```python
from build123d import *

# Parameters (mm, degrees)
SKETCH1_W           = 56
SKETCH1_H           = 100
BOSS_EXTRUDE1_DEPTH = 1.5
SKETCH2_W           = 20
SKETCH2_H           = 5.05
BOSS_EXTRUDE2_DEPTH = 10
SKETCH3_W           = 13.1
SKETCH3_H           = 13.1
CUT_EXTRUDE1_DEPTH  = 112.005866962
BOSS_EXTRUDE3_DEPTH = 5
BOSS_EXTRUDE4_DEPTH = 5
SKETCH6_W           = 7
SKETCH6_H           = 1.5
SKETCH6_W_2         = 1.5
SKETCH6_H_2         = 7
BOSS_EXTRUDE5_DEPTH = 4
SKETCH7_W           = 15
SKETCH7_H           = 1.3
CUT_EXTRUDE2_DEPTH  = 112.005866962
SKETCH8_W           = 13.4
SKETCH8_H           = 8.5
SKETCH8_W_2         = 10
SKETCH8_H_2         = 6
CUT_EXTRUDE3_DEPTH  = 112.005866962
FILLET1_R           = 2
SKETCH9_W           = 15
SKETCH9_H           = 8
BOSS_EXTRUDE6_DEPTH = 1.5
CHAMFER1_SIZE       = 2
SKETCH10_W          = 45
SKETCH10_H          = 59
CUT_EXTRUDE4_DEPTH  = 4
BOSS_EXTRUDE7_DEPTH = 1.5
FILLET2_R           = 1
FILLET3_R           = 0.5


with BuildPart() as part:
    # Sketch1 → Boss-Extrude1 (new body)
    with BuildSketch(Plane.XY):
        with Locations((0, -56.95)):
            Rectangle(SKETCH1_W, SKETCH1_H)
    extrude(amount=BOSS_EXTRUDE1_DEPTH)

    # Sketch2 → Boss-Extrude2 (add)
    with BuildSketch(Plane.XY.offset(1.5)):
        with Locations((-18, -9.475)):
            Rectangle(SKETCH2_W, SKETCH2_H)
        with Locations((18, -9.475)):
            Rectangle(SKETCH2_W, SKETCH2_H)
    extrude(amount=BOSS_EXTRUDE2_DEPTH)

    # Sketch3 → Cut-Extrude1 (cut, through all)
    with BuildSketch(Plane.XY.offset(1.5)):
        with Locations((-16.45, -18.55)):
            Rectangle(SKETCH3_W, SKETCH3_H)
    extrude(amount=-CUT_EXTRUDE1_DEPTH, mode=Mode.SUBTRACT)

    # Sketch4 → Boss-Extrude3 (add)
    with BuildSketch(Plane(origin=(28, 0, 0), x_dir=(0, 0, -1), z_dir=(1, 0, 0))):
        Polygon((-11.5, -12), (-1.5, -12), (-1.5, -22), align=None)
    extrude(amount=-BOSS_EXTRUDE3_DEPTH)

    # Sketch5 → Boss-Extrude4 (add)
    with BuildSketch(Plane.ZY.offset(28)):
        Polygon((1.5, -22), (11.5, -12), (1.5, -12), align=None)
    extrude(amount=-BOSS_EXTRUDE4_DEPTH)

    # Sketch6 → Boss-Extrude5 (add)
    with BuildSketch(Plane.XY.offset(1.5)):
        with Locations((-16.45, -25.85)):
            Rectangle(SKETCH6_W, SKETCH6_H)
        with Locations((-9.15, -18.55)):
            Rectangle(SKETCH6_W_2, SKETCH6_H_2)
    extrude(amount=BOSS_EXTRUDE5_DEPTH)

    # Sketch7 → Cut-Extrude2 (cut, through all)
    with BuildSketch(Plane.XY.offset(1.5)):
        with Locations((0, -28.45)):
            Rectangle(SKETCH7_W, SKETCH7_H)
    extrude(amount=-CUT_EXTRUDE2_DEPTH, mode=Mode.SUBTRACT)

    # Sketch8 → Cut-Extrude3 (cut, through all)
    with BuildSketch(Plane.XY.offset(1.5)):
        with Locations((0, -33.35)):
            Rectangle(SKETCH8_W, SKETCH8_H)
        with Locations((0, -21.8)):
            Rectangle(SKETCH8_W_2, SKETCH8_H_2)
    extrude(amount=-CUT_EXTRUDE3_DEPTH, mode=Mode.SUBTRACT)

    # Fillet1
    fillet1_edges = [part.edges().sort_by_distance(p)[0] for p in [
        (-16.45, -26.6, 1.5),
        (-8.4, -18.55, 1.5),
    ]]
    fillet(fillet1_edges, radius=FILLET1_R)

    # Sketch9 → Boss-Extrude6 (add)
    with BuildSketch(Plane.XY.offset(1.5)):
        with Locations((0, -110.95)):
            Rectangle(SKETCH9_W, SKETCH9_H)
    extrude(amount=-BOSS_EXTRUDE6_DEPTH)

    # Chamfer1
    chamfer1_edges = [part.edges().sort_by_distance(p)[0] for p in [
        (-7.5, -114.95, 0.75),
        (7.5, -114.95, 0.75),
    ]]
    chamfer(chamfer1_edges, length=CHAMFER1_SIZE)

    # Sketch10 → Cut-Extrude4 (cut)
    with BuildSketch(Plane.XY.offset(1.5)):
        with Locations((0, -72.45)):
            Rectangle(SKETCH10_W, SKETCH10_H)
    extrude(amount=-CUT_EXTRUDE4_DEPTH, mode=Mode.SUBTRACT)

    # Sketch11 → Boss-Extrude7 (add)
    with BuildSketch(Plane.XY.offset(1.5)):
        with BuildLine():
            Line((-21.242331765, -42.95), (-22.5, -42.95))
            Line((-22.5, -42.95), (-22.5, -44.598942796))
            Line((-22.5, -44.598942796), (-2.829214626, -70.389528064))
            ThreePointArc((-2.829214626, -70.389528064), (-2.122572116, -69.667072115), (-1.238970121, -69.176629712))
            Line((-1.238970121, -69.176629712), (-21.242331765, -42.95))
        make_face()
        with BuildLine():
            Line((22.5, -42.95), (21.242331765, -42.95))
            Line((21.242331765, -42.95), (1.238970121, -69.176629712))
            ThreePointArc((1.238970121, -69.176629712), (2.122572116, -69.667072115), (2.829214626, -70.389528064))
            Line((2.829214626, -70.389528064), (22.5, -44.598942796))
            Line((22.5, -44.598942796), (22.5, -42.95))
        make_face()
        with BuildLine():
            Line((22.5, -100.301057204), (2.829214626, -74.510471936))
            ThreePointArc((2.829214626, -74.510471936), (2.122572116, -75.232927885), (1.238970121, -75.723370288))
            Line((1.238970121, -75.723370288), (21.242331765, -101.95))
            Line((21.242331765, -101.95), (22.5, -101.95))
            Line((22.5, -101.95), (22.5, -100.301057204))
        make_face()
        with BuildLine():
            Line((-2.829214626, -74.510471936), (-22.5, -100.301057204))
            Line((-22.5, -100.301057204), (-22.5, -101.95))
            Line((-22.5, -101.95), (-21.242331765, -101.95))
            Line((-21.242331765, -101.95), (-1.238970121, -75.723370288))
            ThreePointArc((-1.238970121, -75.723370288), (-2.122572116, -75.232927885), (-2.829214626, -74.510471936))
        make_face()
        with BuildLine():
            Line((-1.257668235, -72.45), (-2.829214626, -70.389528064))
            ThreePointArc((-2.829214626, -70.389528064), (-3.5, -72.45), (-2.829214626, -74.510471936))
            Line((-2.829214626, -74.510471936), (-1.257668235, -72.45))
        make_face()
        with BuildLine():
            Line((0, -70.801057204), (-1.238970121, -69.176629712))
            ThreePointArc((-1.238970121, -69.176629712), (-2.122572116, -69.667072115), (-2.829214626, -70.389528064))
            Line((-2.829214626, -70.389528064), (-1.257668235, -72.45))
            Line((-1.257668235, -72.45), (0, -70.801057204))
        make_face()
        with BuildLine():
            Line((0, -74.098942796), (-1.257668235, -72.45))
            Line((-1.257668235, -72.45), (-2.829214626, -74.510471936))
            ThreePointArc((-2.829214626, -74.510471936), (-2.122572116, -75.232927885), (-1.238970121, -75.723370288))
            Line((-1.238970121, -75.723370288), (0, -74.098942796))
        make_face()
        with BuildLine():
            Line((1.238970121, -75.723370288), (0, -74.098942796))
            Line((0, -74.098942796), (-1.238970121, -75.723370288))
            ThreePointArc((-1.238970121, -75.723370288), (0, -75.95), (1.238970121, -75.723370288))
        make_face()
        with BuildLine():
            Line((2.829214626, -70.389528064), (1.257668235, -72.45))
            Line((1.257668235, -72.45), (2.829214626, -74.510471936))
            ThreePointArc((2.829214626, -74.510471936), (3.328081369, -73.533454846), (3.5, -72.45))
            ThreePointArc((3.5, -72.45), (3.328081369, -71.366545154), (2.829214626, -70.389528064))
        make_face()
        with BuildLine():
            Line((2.829214626, -74.510471936), (1.257668235, -72.45))
            Line((1.257668235, -72.45), (0, -74.098942796))
            Line((0, -74.098942796), (1.238970121, -75.723370288))
            ThreePointArc((1.238970121, -75.723370288), (2.122572116, -75.232927885), (2.829214626, -74.510471936))
        make_face()
        with BuildLine():
            Line((1.238970121, -69.176629712), (0, -70.801057204))
            Line((0, -70.801057204), (1.257668235, -72.45))
            Line((1.257668235, -72.45), (2.829214626, -70.389528064))
            ThreePointArc((2.829214626, -70.389528064), (2.122572116, -69.667072115), (1.238970121, -69.176629712))
        make_face()
        with BuildLine():
            ThreePointArc((1.238970121, -69.176629712), (0, -68.95), (-1.238970121, -69.176629712))
            Line((-1.238970121, -69.176629712), (0, -70.801057204))
            Line((0, -70.801057204), (1.238970121, -69.176629712))
        make_face()
        Polygon((1.257668235, -72.45), (0, -70.801057204), (-1.257668235, -72.45), (0, -74.098942796), align=None)
    extrude(amount=-BOSS_EXTRUDE7_DEPTH)

    # Fillet2
    fillet2_edges = [part.edges().sort_by_distance(p)[0] for p in [
        (-22.5, -100.301057204, 0.75),
        (-21.242331765, -101.95, 0.75),
        (21.242331765, -101.95, 0.75),
        (22.5, -100.301057204, 0.75),
        (22.5, -44.598942796, 0.75),
        (21.242331765, -42.95, 0.75),
        (-21.242331765, -42.95, 0.75),
        (-22.5, -44.598942796, 0.75),
    ]]
    fillet(fillet2_edges, radius=FILLET2_R)

    # Fillet3
    fillet3_edges = [part.edges().sort_by_distance(p)[0] for p in [
        (6.7, -29.1, 0.75),
        (-6.7, -29.1, 0.75),
    ]]
    fillet(fillet3_edges, radius=FILLET3_R)


solid = part.part
```
Input: part model. Units: mm. Frame: model coordinates. A direction names the side the tool comes from. Coordinates: 2 decimals unless noted, no trailing zeros. Write each loop counter-clockwise with the first axis right and the second up, starting at its lowest first coordinate (ties: lowest second). Pieces come first, ordered by that corner, then holes. Notation, with made-up numbers: (-12.5, 17) - (11.5, 17) arc R26 cw to (11.5, 45) - close; hole circle Ø10 at (63, 72). An arc over 180 degrees is marked (long way). Put each result on its own line as item: value. Start each with the question number.
1) Cut plane B-B (x = -17). Return the cut outline in (y, z), plus the area to 3 significant figures.
2) Reachability of faces 4 (the face through (15, -12, 6)), 5 (the face through (25.5, -17.1, 6.4)), 6 (the face through (-9, -15.05, 3)), 7 (the face through (18, -9, 11.5)), 8 (the face through (-11.64, -86.06, 0.76)) from +Z, -Z, +X, -X, +Y, -Y: full face, straight path, thin tool, end or side. Return the list, or none.
3) Contact query for flat-ended pins moving along their axis: pin 1 (0.6 mm diameter, centred on x = -18, z = 4.5, fed in from -Y); pin 2 (1.5 mm diameter, centred on x = 12.5, z = 3, fed in from -Y); pin 3 (1.2 mm diameter, centred on x = -15, z = 1, fed in from -Y); pin 4 (6 mm diameter, centred on x = 3.5, y = -60, fed in from -Z). Output: stop coordinate, or through.
4) Cut plane D-D (y = -51). Return the cut outline in (x, z), plus the area to 3 significant figures.
5) Ray query, L1, parallel to X at y = -14, z = 6.5; L2, parallel to Y at x = -4, z = 1; L3, parallel to Z at x = -12, y = -36. Return the intervals inside material, ascending.
6) Mould query, pull axis Y, two halves, no side actions, for faces 1 (the face through (18, -48, 0)), 2 (the face through (11.64, -58.84, 0.76)), 3 (the face through (6.51, -113.94, 0.76)). Classes: pulls with the +Y half, pulls with the -Y half, needs draft (parallel to the pull), parting line crosses it, or undercut.
7) Cut plane C-C (x = 17). Return the cut outline in (y, z), plus the area to 3 significant figures.
8) Cut plane A-A (z = 7). Return the cut outline in (x, y).
Resolved:
1. outline: (-106.95, 0) - (-101.95, 0) - (-101.95, 1.5) - (-106.95, 1.5) - close; (-96.39, 0) - (-93.09, 0) - (-93.09, 1.5) - (-96.39, 1.5) - close; (-51.81, 0) - (-48.51, 0) - (-48.51, 1.5) - (-51.81, 1.5) - close; (-42.95, 0) - (-25.1, 0) - (-25.1, 5.5) - (-26.6, 5.5) - (-26.6, 3.5) arc R2 cw to (-28.6, 1.5) - (-42.95, 1.5) - close; (-12, 0) - (-6.95, 0) - (-6.95, 11.5) - (-12, 11.5) - close
1. area: 109 mm2
2. face 4: +Z, -Y
2. face 5: +Z, +X, -Y
2. face 6: +Z
2. face 7: +Z, +X, -X, +Y, -Y
2. face 8: +Z, -Z
3. pin 1: stops at y = -26.6
3. pin 2: stops at y = -12
3. pin 3: stops at y = -106.95
3. pin 4: passes through
4. outline: (-28, 0) - (-22.5, 0) - (-22.5, 1.5) - (-28, 1.5) - close; (-17.62, 0) - (-15.1, 0) - (-15.1, 1.5) - (-17.62, 1.5) - close; (15.1, 0) - (17.62, 0) - (17.62, 1.5) - (15.1, 1.5) - close; (22.5, 0) - (28, 0) - (28, 1.5) - (22.5, 1.5) - close
4. area: 24.0 mm2
5. L1: x = -28 to -23, 23 to 28
5. L2: y = -114.95 to -101.95, -79.34 to -76.05, -68.85 to -65.56, -42.95 to -37.6, -27.8 to -24.8, -18.8 to -6.95
5. L3: z = 0 to 1.5
6. face 1: needs draft
6. face 2: undercut
6. face 3: pulls with the -Y half
7. outline: (-106.95, 0) - (-101.95, 0) - (-101.95, 1.5) - (-106.95, 1.5) - close; (-96.39, 0) - (-93.09, 0) - (-93.09, 1.5) - (-96.39, 1.5) - close; (-51.81, 0) - (-48.51, 0) - (-48.51, 1.5) - (-51.81, 1.5) - close; (-42.95, 0) - (-6.95, 0) - (-6.95, 11.5) - (-12, 11.5) - (-12, 1.5) - (-42.95, 1.5) - close
7. area: 122 mm2
8. outline: (-28, -16.5) - (-23, -16.5) - (-23, -12) - (-8, -12) - (-8, -6.95) - (-28, -6.95) - close; (8, -12) - (23, -12) - (23, -16.5) - (28, -16.5) - (28, -6.95) - (8, -6.95) - close
